```python
from build123d import *

# Parameters (mm, degrees)
SKETCH_1_W          = 15
SKETCH_1_H          = 15
SKETCH_1_W_2        = 13
SKETCH_1_H_2        = 13
EXTRUDE_1_DEPTH     = 51
SKETCH_2_R          = 1.45
CUT_EXTRUDE_1_DEPTH = 54.686590505
SKETCH_3_R          = 1.45
CUT_EXTRUDE_2_DEPTH = 54.686590505


with BuildPart() as part:
    # 草图1 → 凸台-拉伸1 (new body)
    with BuildSketch(Plane(origin=(0, 0, 0), x_dir=(0, 0, -1), z_dir=(1, 0, 0))):
        Rectangle(SKETCH_1_W, SKETCH_1_H)
        Rectangle(SKETCH_1_W_2, SKETCH_1_H_2, mode=Mode.SUBTRACT)
    extrude(amount=EXTRUDE_1_DEPTH)

    # 草图2 → 切除-拉伸1 (cut, through all)
    with BuildSketch(Plane(origin=(0, 7.5, 0), x_dir=(1, 0, 0), z_dir=(0, 1, 0))):
        with Locations(Location((7.5, 0, 0), (0, 0, 270))):
            Circle(SKETCH_2_R)
        with Locations(Location((17.5, 0, 0), (0, 0, 270))):
            Circle(SKETCH_2_R)
        with Locations(Location((46, 0, 0), (0, 0, 270))):
            Circle(SKETCH_2_R)
        with Locations(Location((36, 0, 0), (0, 0, 270))):
            Circle(SKETCH_2_R)
    extrude(amount=-CUT_EXTRUDE_1_DEPTH, mode=Mode.SUBTRACT)

    # 草图3 → 切除-拉伸2 (cut, through all)
    with BuildSketch(Plane.XY.offset(7.5)):
        with Locations((5, 0)):
            Circle(SKETCH_3_R)
        with Locations((15, 0)):
            Circle(SKETCH_3_R)
    extrude(amount=-CUT_EXTRUDE_2_DEPTH, mode=Mode.SUBTRACT)


solid = part.part
```
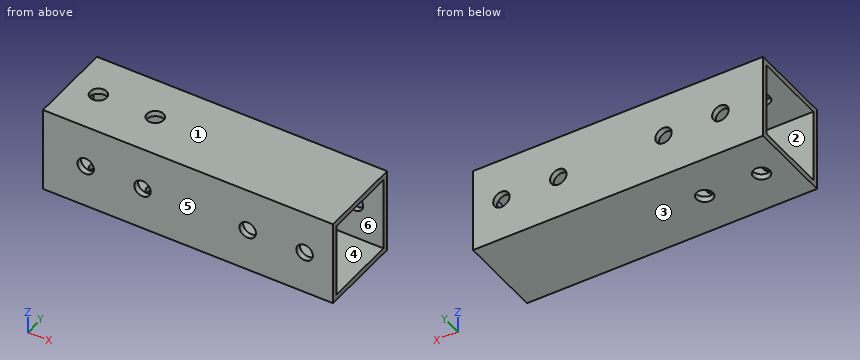
Part model, mm, in its own coordinate system. Face numbers are marked on the shaded views. A direction names the side the tool comes from. Give positions to 0.01 mm unless a question says otherwise; leave off trailing zeros. Order: outer loops, then holes, each group sorted by start corner. A loop starts at its lowest first (then second) coordinate and runs counter-clockwise, first axis right, second up. Notation, with made-up numbers: M 2.5,18 L 6.5,18 A21 cw 6.5,34 Z; hole C 61.25,29 d2. An arc over 180 degrees is marked long. Use a Markdown table: item, result. Add a question column.
(1) Mould opens along Z. For the marked faces 1, 2, 3 and 4 say: +Z half, -Z half, draft (parallel to the pull), parting line (faces both ways), or undercut.
(2) Saw through at C-C, the plane x = 25. Give the cut face in (y, z).
(3) Saw through at D-D, the plane x = 7.5. Give the cut face in (y, z).
(4) Saw through at A-A, the plane y = 2.25. Give the cut face in (x, z), and give its area (3 significant figures).
(5) Probe line 1 along X through (y, z) = (7.05, 0); line 2 along Y through (x, z) = (32, -5.75); line 3 along Y through (x, z) = (15, -6.65). List the from-to ranges inside material, lowest first. Write a range as [from, to].
(6) Drop a flat-ended pin along its axis: P1, Ø2.5, axis at x = 36, z = 0, coming from the +Y side. Give the stop position or say it passes through.
(7) 3-axis set-ups, long thin cutter, end or side, ignore diameter. For the marked faces 5 and 6: which of +Z, -Z, +X, -X, +Y, -Y reach the whole face in a straight line?
Answer key:
| question | item | result |
|---|---|---|
| 1 | face 1 | +Z half |
| 1 | face 2 | undercut |
| 1 | face 3 | -Z half |
| 1 | face 4 | undercut |
| 2 | outline | M -7.5,-7.5 L 7.5,-7.5 L 7.5,7.5 L -7.5,7.5 Z; hole M -6.5,-6.5 L 6.5,-6.5 L 6.5,6.5 L -6.5,6.5 Z |
| 3 | outline | M -7.5,-7.5 L 7.5,-7.5 L 7.5,-1.45 L 6.5,-1.45 L 6.5,-6.5 L -6.5,-6.5 L -6.5,-1.45 L -7.5,-1.45 Z; M -7.5,1.45 L -6.5,1.45 L -6.5,6.5 L 6.5,6.5 L 6.5,1.45 L 7.5,1.45 L 7.5,7.5 L -7.5,7.5 Z |
| 4 | outline | M 0,-7.5 L 51,-7.5 L 51,-6.5 L 0,-6.5 Z; M 0,6.5 L 51,6.5 L 51,7.5 L 0,7.5 Z |
| 4 | area | 102 mm^2 |
| 5 | line 1 | [0, 6.05], [8.95, 16.05], [18.95, 34.55], [37.45, 44.55], [47.45, 51] |
| 5 | line 2 | [-7.5, -6.5], [6.5, 7.5] |
| 5 | line 3 | [-7.5, -1.45], [1.45, 7.5] |
| 6 | P1 | through |
| 7 | face 5 | +Z, -Z, +X, -X, -Y |
| 7 | face 6 | +X, -X |
